CAD build for the part. Positions are in the model's coordinates, mm. Give positions to 0.01 mm unless a question says otherwise; leave off trailing zeros. Order: outer loops, then holes, each group sorted by start corner. A loop starts at its lowest first (then second) coordinate and runs counter-clockwise, first axis right, second up.
Item 1: Wall check: L1, parallel to Y at x = 0, z = 3.75; L2, parallel to X at y = -19, z = 7.75; L3, parallel to X at y = 19.5, z = 3.25. Give the ranges that are in metal, low to high.
Item 2: Two-plate mould, pull along Y, no slides. Class faces 1 (the flat face through (0, 0, 0)), 2 (the flat face through (0, 30, 5)), 3 (the cylindrical face through (1.13, 21.77, 4.93)): released by +Y, released by -Y, zero draft, split by the parting line, or undercut.
Item 3: Flat gauge pins, fed straight in: P1, Ø5, axis at y = -4, z = 9, coming from the +X side; P2, Ø1, axis at y = 1.5, z = 3.5, coming from the -X side; P3, Ø1, axis at y = 8.5, z = 3, coming from the -X side. Where does each tip first touch, or does it go through?
Item 4: Band-saw the part on D-D on y = 6. Give the cut face in (x, z).
Item 5: Band-saw the part on A-A on x = 0. Give the cut face in (y, z), plus the area to 3 significant figures.
Item 6: Band-saw the part on B-B on y = -20. Give the cut face in (x, z), plus the area to 3 significant figures.
Item 7: Band-saw the part on C-C on z = 5.5. Give the cut face in (x, y), plus the area to 3 significant figures.
```python
from build123d import *

# Parameters (mm, degrees)
IZIM1_W                     = 43.801650212
IZIM1_H                     = 60
IZIM1_R                     = 2.1
Y_KSEKLIK_EKSTR_ZYON1_DEPTH = 10
KES_EKSTR_ZYON1_DEPTH       = 81


with BuildPart() as part:
    # Çizim1 → Yükseklik-Ekstrüzyon1 (new body)
    with BuildSketch(Plane.XY):
        Rectangle(IZIM1_W, IZIM1_H)
        with Locations((0, -20)):
            Circle(IZIM1_R, mode=Mode.SUBTRACT)
        with Locations((0, 20)):
            Circle(IZIM1_R, mode=Mode.SUBTRACT)
    extrude(amount=Y_KSEKLIK_EKSTR_ZYON1_DEPTH)

    # Çizim2 → Kes-Ekstrüzyon1 (cut)
    with BuildSketch(Plane(origin=(0, 30, 0), x_dir=(1, 0, 0), z_dir=(0, 1, 0))):
        Polygon((-15.608960187, 10.547911998), (-27.517863297, 10.547911998), (-27.517863297, -12.148896601), (-18.937760084, -10.469303395), align=None)
        Polygon((27.517863297, -12.148896601), (18.937760084, -10.469303395), (15.608960187, 10.547911998), (27.517863297, 10.547911998), align=None)
    extrude(amount=-KES_EKSTR_ZYON1_DEPTH, mode=Mode.SUBTRACT)


solid = part.part
```
The answers:
1. L1: y = -30 to -22.1, -17.9 to 17.9, 22.1 to 30
1. L2: x = -18.51 to -1.85, 1.85 to 18.51
1. L3: x = -17.79 to -2.04, 2.04 to 17.79
2. face 1: zero draft
2. face 2: released by +Y
2. face 3: undercut
3. P1: stops at x = 18.86
3. P2: stops at x = -17.91
3. P3: stops at x = -17.83
4. outline: (-18.86, 10) - (-17.28, 0) - (17.28, 0) - (18.86, 10) - close
5. outline: (-30, 0) - (-22.1, 0) - (-22.1, 10) - (-30, 10) - close; (-17.9, 0) - (17.9, 0) - (17.9, 10) - (-17.9, 10) - close; (22.1, 0) - (30, 0) - (30, 10) - (22.1, 10) - close
5. area: 516 mm2
6. outline: (-18.86, 10) - (-17.28, 0) - (-2.1, 0) - (-2.1, 10) - close; (2.1, 0) - (17.28, 0) - (18.86, 10) - (2.1, 10) - close
6. area: 319 mm2
7. outline: (-18.15, -30) - (18.15, -30) - (18.15, 30) - (-18.15, 30) - close; hole circle Ø4.2 at (0, -20); hole circle Ø4.2 at (0, 20)
7. area: 2,150 mm2
